Part model, mm, in its own coordinate system. Face numbers are marked on the shaded views. Give positions to 0.01 mm unless a question says otherwise; leave off trailing zeros. Write each loop counter-clockwise with the first axis right and the second up, starting at its lowest first coordinate (ties: lowest second). Pieces come first, ordered by that corner, then holes.
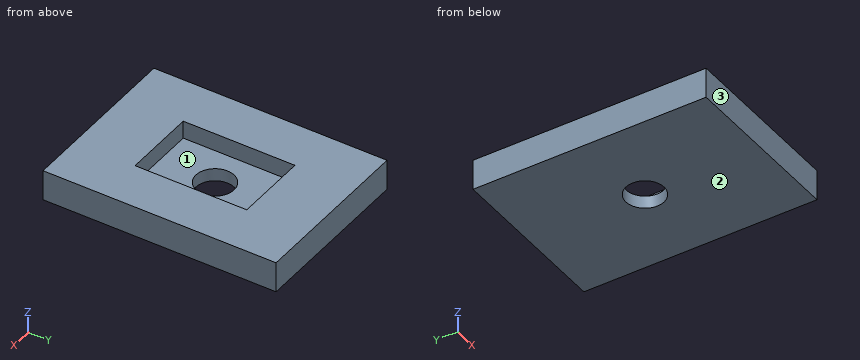
Autodesk Inventor part; units mm, degrees
ref_plane "YZ Plane" through (0, 0, 0) normal (1, 0, 0) x (0, 1, 0)
ref_plane "XZ Plane" through (0, 0, 0) normal (0, 1, 0) x (-1, 0, 0)
ref_plane "XY Plane" through (0, 0, 0) normal (0, 0, 1) x (1, 0, 0)
ref_plane "Arbeitsebene1" through (0, 0, 0) normal (0, 0, 1) x (1, 0, 0)
sketch "Skizze1" plane through (0, 0, 0) normal (0, 0, 1) x (1, 0, 0)
  line L0 (-28.4, 40.9) -> (28.4, 40.9)
  line L1 (28.4, 40.9) -> (28.4, -40.9)
  line L2 (28.4, -40.9) -> (-28.4, -40.9)
  line L3 (-28.4, -40.9) -> (-28.4, 40.9)
  line L4 (-33.4, 45.9) -> (-33.4, -45.9)
  line L5 (-33.4, -45.9) -> (33.4, -45.9)
  line L6 (33.4, -45.9) -> (33.4, 45.9)
  line L7 (33.4, 45.9) -> (-33.4, 45.9)
  line L8 (-28.4, 40.9) -> (28.4, 40.9)
  line L9 (28.4, 40.9) -> (28.4, -40.9)
  line L10 (28.4, -40.9) -> (-28.4, -40.9)
  line L11 (-28.4, -40.9) -> (-28.4, 40.9)
  line L12 (-33.4, 45.9) -> (-33.4, -45.9)
  line L13 (-33.4, -45.9) -> (33.4, -45.9)
  line L14 (33.4, -45.9) -> (33.4, 45.9)
  line L15 (33.4, 45.9) -> (-33.4, 45.9)
  point P0 (0, 0)
extrude "Extrusion1" add sketch "Skizze1" along normal blind 5 contours L0 L1 L2 L3 | L7 L6 L5 L4
sketch "Skizze2" plane through (0, 0, 5) normal (0, 0, 1) x (1, 0, 0)
  circle A0 centre (0, 0) radius 7.5
  dimension "d2" = 15
extrude "Extrusion2" cut sketch "Skizze2" against normal up to next
sketch "Skizze3" plane through (0, 0, 5) normal (0, 0, 1) x (1, 0, 0)
  line L0 (-33.4, 45.9) -> (-33.4, -45.9)
  line L1 (-33.4, -45.9) -> (33.4, -45.9)
  line L2 (33.4, -45.9) -> (33.4, 45.9)
  line L3 (33.4, 45.9) -> (-33.4, 45.9)
  line L4 (-14.5, 22) -> (14.5, 22)
  line L5 (14.5, 22) -> (14.5, -22)
  line L6 (14.5, -22) -> (-14.5, -22)
  line L7 (-14.5, -22) -> (-14.5, 22)
  line L8 (0, -64.26) -> (0, 64.26)
  line L9 (-46.76, 0) -> (46.76, 0)
  dimension "d9" = 29
  dimension "d10" = 44
extrude "Extrusion4" add sketch "Skizze3" along normal blind 7 contours L3 L8 L4 L7 L9 L0 | L9 L7 L6 L8 L1 L0 | L3 L2 L9 L5 L4 L8 | L8 L6 L5 L9 L2 L1
properties part number "InlayOben" material "Gummi, Silikon"
1) Two-plate mould, pull along Y, no slides. Class the marked faces 1, 2 and 3: +Y half, -Y half, draft (parallel to the pull), parting line (faces both ways), or undercut.
Answers follow:
face 1: undercut
face 2: draft
face 3: -Y half
2) Pin check, flat tip, straight feed: pin 1 Ø19.5 at (x, y) = (0, 0) entering from +Z. Stop position of the tip, or through.
Answers follow:
pin 1: stops at z = 5
3) Saw through at B-B, the plane x = 0. Write the cut outline in (y, z), then the cut area to 3 significant figures.
Answers follow:
outline: (-45.9, 0) - (-7.5, 0) - (-7.5, 5) - (-22, 5) - (-22, 12) - (-45.9, 12) - close; (7.5, 0) - (45.9, 0) - (45.9, 12) - (22, 12) - (22, 5) - (7.5, 5) - close
area: 719 mm2
4) Saw through at C-C, the plane y = 14.5. Write the cut outline in (x, z).
Answers follow:
outline: (-33.4, 0) - (33.4, 0) - (33.4, 12) - (14.5, 12) - (14.5, 5) - (-14.5, 5) - (-14.5, 12) - (-33.4, 12) - close
5) Saw through at A-A, the plane y = 0. Write the cut outline in (x, z).
Answers follow:
outline: (-33.4, 0) - (-7.5, 0) - (-7.5, 5) - (-14.5, 5) - (-14.5, 12) - (-33.4, 12) - close; (7.5, 0) - (33.4, 0) - (33.4, 12) - (14.5, 12) - (14.5, 5) - (7.5, 5) - close
6) Wall check: L1, parallel to X at y = -6.5, z = 5.75; L2, parallel to Y at x = -14, z = 5.25; L3, parallel to Y at x = 0, z = 3.25. Give the ranges that are in metal, low to high.
Answers follow:
L1: x = -33.4 to -14.5, 14.5 to 33.4
L2: y = -45.9 to -22, 22 to 45.9
L3: y = -45.9 to -7.5, 7.5 to 45.9
